Geometry check sheet. Reference: the model listing, model coordinates, mm. Face numbers are marked on the shaded views. Give positions to 0.01 mm unless a question says otherwise; leave off trailing zeros. Write each loop counter-clockwise with the first axis right and the second up, starting at its lowest first coordinate (ties: lowest second). Pieces come first, ordered by that corner, then holes. Notation, with made-up numbers: (5.5, 29) - (32.5, 29) arc R6 cw to (32.5, 40) - close; hole circle Ø6 at (56, -27.5). An arc over 180 degrees is marked (long way). Use a Markdown table: item, result.
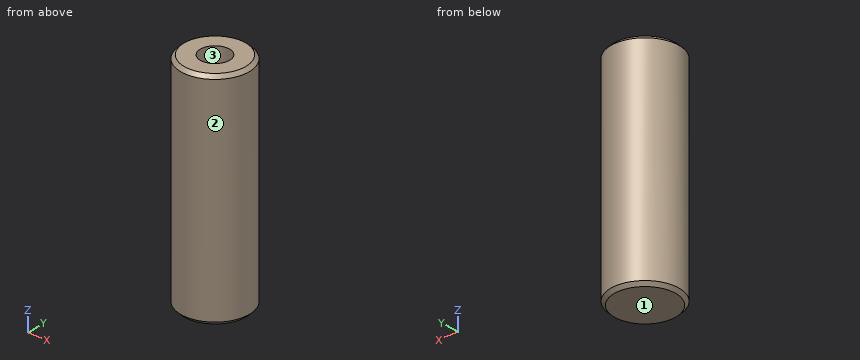
```python
from build123d import *

# Parameters (mm, degrees)
F0_R     = 15.7734
F1_DEPTH = 101.6
F3_D     = 13.49248
F3_DEPTH = 32.3272658
F3_TIP   = 4.0535499425
F4_SIZE  = 1.5875


with BuildPart() as f1:
    # F0 (on Top) → F1 (new body)
    with BuildSketch(Plane.XY):
        with Locations((-36.8766486645, 14.1249885783)):
            Circle(F0_R)
    extrude(amount=F1_DEPTH)

    # F3
    with Locations(Plane.XY.offset(101.6)):
        with Locations((-36.8766486645, 14.1249885783)):
            Hole(F3_D / 2, depth=F3_DEPTH)
            with Locations((0, 0, -(F3_DEPTH + F3_TIP / 2))):  # 118° drill point
                Cone(0, F3_D / 2, F3_TIP, mode=Mode.SUBTRACT)

    # F4
    f4_edges = [f1.edges().sort_by_distance(p)[0] for p in [
        (-52.650049, 14.124989, 0),
        (-52.650049, 14.124989, 101.6),
    ]]
    chamfer(f4_edges, length=F4_SIZE)


solid = f1.part
```
1) Section check B-B on z = 30. Record the boundary of the cut face in (x, y), then the cut area to 3 significant figures.
Working result:
| item | result |
|---|---|
| outline | circle Ø31.55 at (-36.88, 14.12) |
| area | 782 mm² |
2) Material ranges on L1, parallel to X at y = 14, z = 20.5; L2, parallel to Y at x = -39.5, z = 27.5; L3, parallel to Y at x = -44, z = 84, recorded low to high. Write a range as from..to.
Working result:
| item | result |
|---|---|
| L1 | x = -52.65..-21.1 |
| L2 | y = -1.43..29.68 |
| L3 | y = 0.05..28.2 |
3) Mould release check, pull along Y, two halves, no side actions. Record for the marked faces 1, 2 and 3: pulls with the +Y half, pulls with the -Y half, needs draft (parallel to the pull), parting line crosses it, or undercut.
Working result:
| item | result |
|---|---|
| face 1 | needs draft |
| face 2 | parting line crosses it |
| face 3 | undercut |
4) Depth check by flat-ended pin: P1, Ø2, axis at x = -44, z = 91, coming from the +Y side; P2, Ø1.5, axis at x = -42.5, z = 58.5, coming from the -Y side; P3, Ø4, axis at x = -25, z = 16.5, coming from the +Y side. Enter the tip coordinate at first touch or a pass-through.
Working result:
| item | result |
|---|---|
| P1 | stops at y = 28.66 |
| P2 | stops at y = -0.88 |
| P3 | stops at y = 26.42 |
5) Section check A-A on z = 89. Record the boundary of the cut face in (x, y), then the cut area to 3 significant figures.
Working result:
| item | result |
|---|---|
| outline | circle Ø31.55 at (-36.88, 14.12); hole circle Ø13.49 at (-36.88, 14.12) |
| area | 639 mm² |
